Print and shaded views of the part. All mm, measured from the part's lowest x, y and z. Round coordinates to 2 decimals unless told otherwise and drop trailing zeros. Write each loop counter-clockwise with the first axis right and the second up, starting at its lowest first coordinate (ties: lowest second). Pieces come first, ordered by that corner, then holes. Notation, with made-up numbers: (26.25, -31.5) -> (36.25, -31.5) arc R18 cw to (36.25, -14.5) -> close; hole circle Ø1 at (-27, 13). An arc over 180 degrees is marked (long way). Use CSV: the item, a comma, the result in double quotes. Start each with the question number.
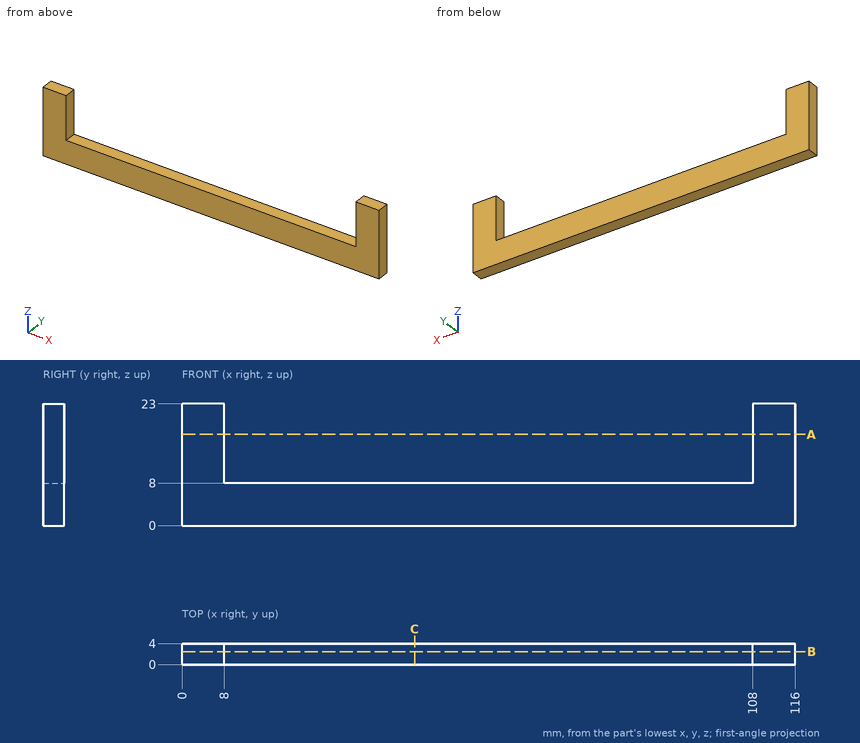
1. Band-saw the part on B-B (y = 2.45). List the corners of the cut face in (x, z), then the cut area to 3 significant figures.
2. Band-saw the part on C-C (x = 44). List the corners of the cut face in (y, z), then the cut area to 3 significant figures.
3. Drill centre lines: line 1 along X through (y, z) = (1.05, 12.5); line 2 along Z through (x, y) = (41.5, 2.5). Where is each one in solid material? Low to high. Write a range as [from, to].
4. Band-saw the part on A-A (z = 17.25). List the corners of the cut face in (x, y).
Answers below:
1,outline,"(0, 0) -> (116, 0) -> (116, 23) -> (108, 23) -> (108, 8) -> (8, 8) -> (8, 23) -> (0, 23) -> close"
1,area,"1,170 mm^2"
2,outline,"(0, 0) -> (4, 0) -> (4, 8) -> (0, 8) -> close"
2,area,"32.0 mm^2"
3,line 1,"x = [0, 8], [108, 116]"
3,line 2,"z = [0, 8]"
4,outline,"(0, 0) -> (8, 0) -> (8, 4) -> (0, 4) -> close; (108, 0) -> (116, 0) -> (116, 4) -> (108, 4) -> close"
